Source: CAD feature listing. Evaluate the final solid. Frame: model axes, mm. A direction names the side the tool comes from. Round coordinates to 2 decimals unless told otherwise and drop trailing zeros. Order: outer loops, then holes, each group sorted by start corner. A loop starts at its lowest first (then second) coordinate and runs counter-clockwise, first axis right, second up. Notation, with made-up numbers: (11.5, -14) -> (31.5, -14) arc R17 cw to (31.5, 15) -> close; hole circle Ø4 at (24.25, 71.25). An arc over 180 degrees is marked (long way). One line per item, written item: value. Start each with the question number.
1) Section C-C (z = 2.75). Return the cut outline in (x, y), and give its area (3 significant figures).
2) Mould query, pull axis Y, two halves, no side actions, for faces 3 (the face through (-0.71, -10.84, 3.22)), 4 (the face through (-0.7, -5.5, 0)), 5 (the face through (1, 5.08, 3)). Classes: pulls with the +Y half, pulls with the -Y half, needs draft (parallel to the pull), parting line crosses it, or undercut.
3) Reachability of faces 1 (the face through (43.18, -0.11, 3.13)), 2 (the face through (48.94, -0.18, 3.22)) from +Z, -Z, +X, -X, +Y, -Y: full face, straight path, thin tool, end or side. Return the list, or none.
4) Ray query, L1, parallel to Y at x = 20.5, z = 4.5; L2, parallel to Y at x = -21, z = 1.75; L3, parallel to X at y = -0.25, z = 2.5. Return the intervals inside material, ascending.
5) Pin query (flat end, axial travel): P1, Ø3, axis at x = 13, z = 2.5, coming from the -Y side; P2, Ø3, axis at x = 15.5, z = 4, coming from the +Y side; P3, Ø3, axis at y = -4.5, z = 4.5, coming from the +X side. Return the tip coordinate at first contact, or that it passes through.
```python
from build123d import *

# Parameters (mm, degrees)
F0_W     = 101.6
F0_H     = 25.4
F1_DEPTH = 6.35
F2_SIZE2 = 3.666164
F2_SIZE  = 6.34999
F4_DEPTH = 42.2284360975


# Not quite as in the source:
# - a fillet or chamfer is up to 0.001 mm smaller than in the source, because OpenCascade refuses the exact size


with BuildPart() as f1:
    # F0 (on Top) → F1 (new body)
    with BuildSketch(Plane.XY):
        Rectangle(F0_W, F0_H)
    extrude(amount=F1_DEPTH)

    # F2 (size 6.35 and 3.6661742094 in the source; OpenCascade refuses exactly that, so slightly less here)
    f2_edges = [f1.edges().sort_by_distance(p)[0] for p in [
        (0, 12.7, 6.35),
        (-50.8, 0, 6.35),
        (0, -12.7, 6.35),
        (50.8, 0, 6.35),
    ]]
    chamfer(f2_edges, length=F2_SIZE, length2=F2_SIZE2)

    # F3 (on face) → F4 (cut)
    with BuildSketch(Plane.XY):
        with BuildLine():
            ThreePointArc((-38.1, 5.08), (-43.18, 0), (-38.1, -5.08))
            Line((-38.1, -5.08), (38.1, -5.08))
            ThreePointArc((38.1, -5.08), (43.18, 0), (38.1, 5.08))
            Line((38.1, 5.08), (-38.1, 5.08))
        make_face()
    extrude(amount=F4_DEPTH, mode=Mode.SUBTRACT)


solid = f1.part
```
Findings:
1. outline: (-49.21, -11.11) -> (49.21, -11.11) -> (49.21, 11.11) -> (-49.21, 11.11) -> close; hole (-38.1, -5.08) -> (38.1, -5.08) arc R5.08 ccw to (38.1, 5.08) -> (-38.1, 5.08) arc R5.08 ccw to start
1. area: 1,330 mm2
2. face 3: pulls with the -Y half
2. face 4: needs draft
2. face 5: undercut
3. face 1: +Z, -Z
3. face 2: +Z, +X, +Y, -Y
4. L1: -10.1 to -5.08, 5.08 to 10.1
4. L2: -11.69 to -5.08, 5.08 to 11.69
4. L3: -49.36 to -43.17, 43.17 to 49.36
5. P1: y = -12.12
5. P2: y = 11.26
5. P3: x = 49.07
